The listing builds one solid part. Answer for the finished solid, in the listing's coordinates (mm). Coordinates: 2 decimals unless noted, no trailing zeros. Loops run counter-clockwise (first coordinate to the right, second up) from the corner with the lowest first, then second, coordinate; pieces in that order, holes last. Notation, with made-up numbers: (-9, 56.5) - (-1, 56.5) arc R22 ccw to (-1, 77.5) - close; hole circle Ø3 at (60, 22.5). An arc over 180 degrees is marked (long way). Return JSON: item names as keys, results as strings. Group by question number.
1. Each of these flat-tipped pins is pushed along its axis until it touches: P1, Ø18, axis at x = 80.06, y = 104.27, coming from the -Z side; P2, Ø23, axis at x = 26.06, y = 104.27, coming from the +Z side. Where does it stop, or does it pass through?
2. Section B-B (z = 7.25) is taken. State how many separate pieces and enclosed holes the cut face has, and give its area (3 significant figures).
3. Section D-D (x = 156) is taken. Write down the section's boundary in (y, z), and give its area (3 significant figures).
4. Find the intervals of material crossed by line 1 along Y through (x, z) = (80.5, 1.75); line 2 along Y through (x, z) = (134, 11.25); line 3 along X through (y, z) = (-1, 6.5), in increasing order.
5. Section C-C (y = -26.5) is taken. Write down the section's boundary in (x, z), and give its area (3 significant figures).
6. Section A-A (x = 24.5) is taken. Write down the section's boundary in (y, z), and give its area (3 significant figures).
```python
from build123d import *

# Parameters (mm, degrees)
F0_W     = 275
F0_H     = 175
F1_DEPTH = 12
F2_R     = 25.4
F2_R_2   = 10
F2_R_3   = 26
F3_DEPTH = 7
F4_DEPTH = 25


with BuildPart() as f1:
    # F0 (on Top) → F1 (new body)
    with BuildSketch(Plane.XY):
        with Locations((79.5600198209, 48.7740390003)):
            Rectangle(F0_W, F0_H)
    extrude(amount=F1_DEPTH)

    # F2 (on face) → F3 (cut)
    with BuildSketch(Plane.XY.offset(12)):
        with Locations((-27.9399801791, 104.2740390003)):
            Circle(F2_R)
        with Locations((-27.9399801791, 104.2740390003)):
            Circle(F2_R_2, mode=Mode.SUBTRACT)
        with Locations((-27.9399801791, 48.7740390003)):
            Circle(F2_R)
        with Locations((-27.9399801791, 48.7740390003)):
            Circle(F2_R_2, mode=Mode.SUBTRACT)
        with Locations((-27.9399801791, -6.7259609997)):
            Circle(F2_R_3)
        with Locations((-27.9399801791, -6.7259609997)):
            Circle(F2_R_2, mode=Mode.SUBTRACT)
        with Locations((26.0600198209, -6.7259609997)):
            Circle(F2_R_3)
        with Locations((26.0600198209, -6.7259609997)):
            Circle(F2_R_2, mode=Mode.SUBTRACT)
        with Locations((26.0600198209, 48.7740390003)):
            Circle(F2_R)
        with Locations((26.0600198209, 48.7740390003)):
            Circle(F2_R_2, mode=Mode.SUBTRACT)
        with Locations((26.0600198209, 104.2740390003)):
            Circle(F2_R)
        with Locations((26.0600198209, 104.2740390003)):
            Circle(F2_R_2, mode=Mode.SUBTRACT)
        with Locations((80.0600198209, 104.2740390003)):
            Circle(F2_R)
        with Locations((80.0600198209, 104.2740390003)):
            Circle(F2_R_2, mode=Mode.SUBTRACT)
        with Locations((80.0600198209, 48.7740390003)):
            Circle(F2_R)
        with Locations((80.0600198209, 48.7740390003)):
            Circle(F2_R_2, mode=Mode.SUBTRACT)
        with Locations((80.0600198209, -6.7259609997)):
            Circle(F2_R_3)
        with Locations((80.0600198209, -6.7259609997)):
            Circle(F2_R_2, mode=Mode.SUBTRACT)
        with Locations((134.0600198209, -6.7259608768)):
            Circle(F2_R_3)
        with Locations((134.0600198209, -6.7259608768)):
            Circle(F2_R_2, mode=Mode.SUBTRACT)
        with Locations((134.0600198209, 48.7740391232)):
            Circle(F2_R)
        with Locations((134.0600198209, 48.7740391232)):
            Circle(F2_R_2, mode=Mode.SUBTRACT)
        with Locations((134.0600198209, 104.2740391232)):
            Circle(F2_R)
        with Locations((134.0600198209, 104.2740391232)):
            Circle(F2_R_2, mode=Mode.SUBTRACT)
        with Locations((188.0600198209, 104.2740390003)):
            Circle(F2_R)
        with Locations((188.0600198209, 104.2740390003)):
            Circle(F2_R_2, mode=Mode.SUBTRACT)
        with Locations((188.0600198209, 48.7740390003)):
            Circle(F2_R)
        with Locations((188.0600198209, 48.7740390003)):
            Circle(F2_R_2, mode=Mode.SUBTRACT)
        with Locations((188.0600198209, -6.7259609997)):
            Circle(F2_R_3)
        with Locations((188.0600198209, -6.7259609997)):
            Circle(F2_R_2, mode=Mode.SUBTRACT)
    extrude(amount=-F3_DEPTH, mode=Mode.SUBTRACT)

    # F4 (cut): faces of the model
    f4_faces = [f1.faces().sort_by_distance(p)[0] for p in [
        (-27.9399801791, 104.2740390003, 12),
        (26.0600198209, 104.2740390003, 12),
        (80.0600198209, 104.2740390003, 12),
        (134.0600198209, 104.2740391232, 12),
        (188.0600198209, 104.2740390003, 12),
        (188.0600198209, 48.7740390003, 12),
        (134.0600198209, 48.7740391232, 12),
        (80.0600198209, 48.7740390003, 12),
        (26.0600198209, 48.7740390003, 12),
        (-27.9399801791, 48.7740390003, 12),
        (-27.9399801791, -6.7259609997, 12),
        (26.0600198209, -6.7259609997, 12),
        (80.0600198209, -6.7259609997, 12),
        (134.0600198209, -6.7259608768, 12),
        (188.0600198209, -6.7259609997, 12),
    ]]
    extrude(f4_faces, amount=-F4_DEPTH, mode=Mode.SUBTRACT)


solid = f1.part
```
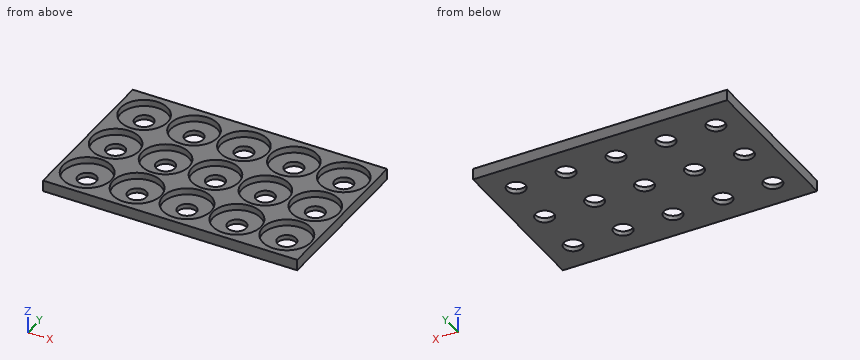
The answers:
{
 "1": {"P1": "passes through", "P2": "stops at z = 5"},
 "2": {"separate pieces": "1", "enclosed holes": "15", "area": "17,200 mm2"},
 "3": {"outline": "(-38.73, 0) - (136.27, 0) - (136.27, 12) - (117.07, 12) - (117.07, 5) - (91.48, 5) - (91.48, 12) - (61.57, 12) - (61.57, 5) - (35.98, 5) - (35.98, 12) - (7.23, 12) - (7.23, 5) - (-20.68, 5) - (-20.68, 12) - (-38.73, 12) - close", "area": "1,550 mm2"},
 "4": {"line 1": "y = -38.73 to -16.72, 3.26 to 38.78, 58.76 to 94.28, 114.26 to 136.27", "line 2": "y = -38.73 to -32.73, 19.27 to 23.37, 74.17 to 78.87, 129.67 to 136.27", "line 3": "x = -57.94 to -53.3, -2.58 to 0.7, 51.42 to 54.7, 105.42 to 108.7, 159.42 to 162.7, 213.42 to 217.06"},
 "5": {"outline": "(-57.94, 0) - (217.06, 0) - (217.06, 12) - (204.94, 12) - (204.94, 5) - (171.18, 5) - (171.18, 12) - (150.94, 12) - (150.94, 5) - (117.18, 5) - (117.18, 12) - (96.94, 12) - (96.94, 5) - (63.18, 5) - (63.18, 12) - (42.94, 12) - (42.94, 5) - (9.18, 5) - (9.18, 12) - (-11.06, 12) - (-11.06, 5) - (-44.82, 5) - (-44.82, 12) - (-57.94, 12) - close", "area": "2,120 mm2"},
 "6": {"outline": "(-38.73, 0) - (-16.6, 0) - (-16.6, 5) - (-32.68, 5) - (-32.68, 12) - (-38.73, 12) - close; (3.15, 0) - (38.9, 0) - (38.9, 5) - (23.42, 5) - (23.42, 12) - (19.23, 12) - (19.23, 5) - (3.15, 5) - close; (58.65, 0) - (94.4, 0) - (94.4, 5) - (78.92, 5) - (78.92, 12) - (74.13, 12) - (74.13, 5) - (58.65, 5) - close; (114.15, 0) - (136.27, 0) - (136.27, 12) - (129.63, 12) - (129.63, 5) - (114.15, 5) - close", "area": "730 mm2"}
}
